The listing builds one solid part. Answer for the finished solid, in the listing's coordinates (mm). Face numbers are marked on the shaded views. Round coordinates to 2 decimals unless told otherwise and drop trailing zeros. Order: outer loops, then holes, each group sorted by start corner. A loop starts at its lowest first (then second) coordinate and runs counter-clockwise, first axis right, second up. Notation, with made-up numbers: M 53,55 L 108,55 A26 ccw 108,91 Z; hole C -23.5,4 d4. An arc over 180 degrees is marked long. Write item = value, one per line. Start each with the question number.
(1) Each of these flat-tipped pins is pushed along its axis until it touches: pin 1 (1.5 mm diameter, centred on y = 3.5, z = -1.5, fed in from -X); pin 2 (6 mm diameter, centred on x = 17.5, y = 17.5, fed in from -Z). Where does it stop, or does it pass through?
(2) For a pull along Y with two mould halves and no side action, classify the marked faces 1, 2 and 3 as released by +Y, released by -Y, zero draft, split by the parting line, or undercut.
(3) A cutting plane is placed at C-C, the plane x = 18.5. Count the separate pieces of the cut face and the enclosed holes in it, and give its area (3 significant figures).
(4) A cutting plane is placed at A-A, the plane x = 0. Determine the outline of the cut face in (y, z), and give its area (4 significant figures).
(5) Straight lines are drawn through the part: probe 1 along X at (y, z) = (-17.5, 0.5); probe 2 along Y at (x, z) = (0, 1.25). For each, find the intervals that lie inside material, in ascending order. Write a range as from..to.
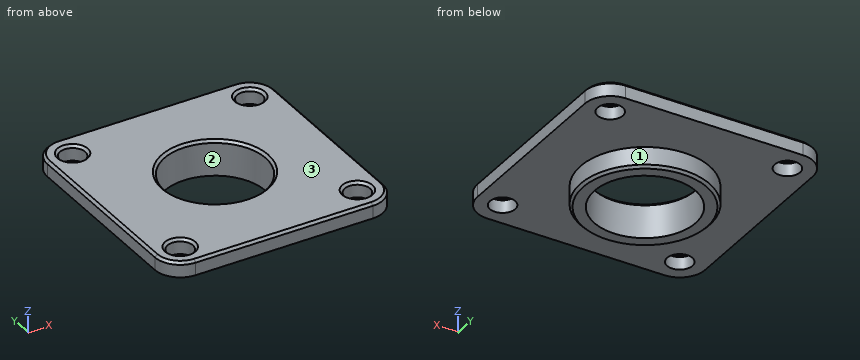
Solid Edge part; units mm, degrees
sketch "Sketch1" plane through (0, 0, 0) normal (0, 0, 1) x (1, 0, 0)
  line L0 (-22.5, 22.5) -> (-22.5, -22.5)
  line L1 (-22.5, -22.5) -> (22.5, -22.5)
  line L2 (22.5, -22.5) -> (22.5, 22.5)
  line L3 (22.5, 22.5) -> (-22.5, 22.5)
  circle A0 centre (0, 0) radius 10
extrude "Extrusionsausprägung_22" add sketch "Sketch1" along normal blind 3
sketch "Sketch2" plane through (0, 0, 0) normal (0, 0, -1) x (1, 0, 0)
  circle A0 centre (0, 0) radius 12.75
  circle A1 centre (0, 0) radius 10
extrude "Extrusionsausprägung_23" add sketch "Sketch2" along normal blind 4
hole "Bohrung_12" at (17.5, -17.5, 3) direction (0, 0, -1) diameter 5 end up to next
hole "Hole1" at (-17.5, -17.5, 3) direction (0, 0, -1) diameter 5 end up to next
hole "Hole2" at (-17.5, 17.5, 3) direction (0, 0, -1) diameter 5 end up to next
hole "Hole3" at (17.5, 17.5, 3) direction (0, 0, -1) diameter 5 end up to next
fillet "Verrundung_18" radius 5 4 edges at (-22.5, -22.5, 1.5) (22.5, -22.5, 1.5) (-22.5, 22.5, 1.5) (22.5, 22.5, 1.5)
chamfer "Fase_11" distance 0.5 angle 45 13 edges at (20, 17.5, 3) (-15, 17.5, 3) (-15, -17.5, 3) (20, -17.5, 3) (-10, 0, 3) (22.5, 0, 3) (21.0355, 21.0355, 3) (0, 22.5, 3) (-21.0355, 21.0355, 3) (-22.5, 0, 3) (-21.0355, -21.0355, 3) (0, -22.5, 3) (21.0355, -21.0355, 3)
chamfer "Fase_12" distance 0.5 angle 45 1 edges at (-12.75, 0, -4)
Reported:
q1.pin_1 = -12.45
q1.pin_2 = 0
q2.face_1 = split by the parting line
q2.face_2 = undercut
q2.face_3 = zero draft
q3.separate_pieces = 3
q3.enclosed_holes = 0
q3.area = 106 mm²
q4.outline = M -22.5,0 L -12.75,0 L -12.75,-3.5 L -12.25,-4 L -10,-4 L -10,2.5 L -10.5,3 L -22,3 L -22.5,2.5 Z; M 10,-4 L 12.25,-4 L 12.75,-3.5 L 12.75,0 L 22.5,0 L 22.5,2.5 L 22,3 L 10.5,3 L 10,2.5 Z
q4.area = 96.25 mm²
q5.probe_1 = -22.5..-20, -15..15, 20..22.5
q5.probe_2 = -22.5..-10, 10..22.5
